Drawing for the job (mm, zero at the part's lowest x, y, z). Round coordinates to 2 decimals unless told otherwise and drop trailing zeros. Write each loop counter-clockwise with the first axis right and the second up, starting at its lowest first coordinate (ties: lowest second). Pieces come first, ordered by that corner, then holes. Notation, with made-up numbers: (13.5, 2) - (66.5, 2) arc R30 ccw to (66.5, 27) - close; hole circle Ø8 at (44, 63). An arc over 180 degrees is marked (long way). One line per question, with ' | ' between items.
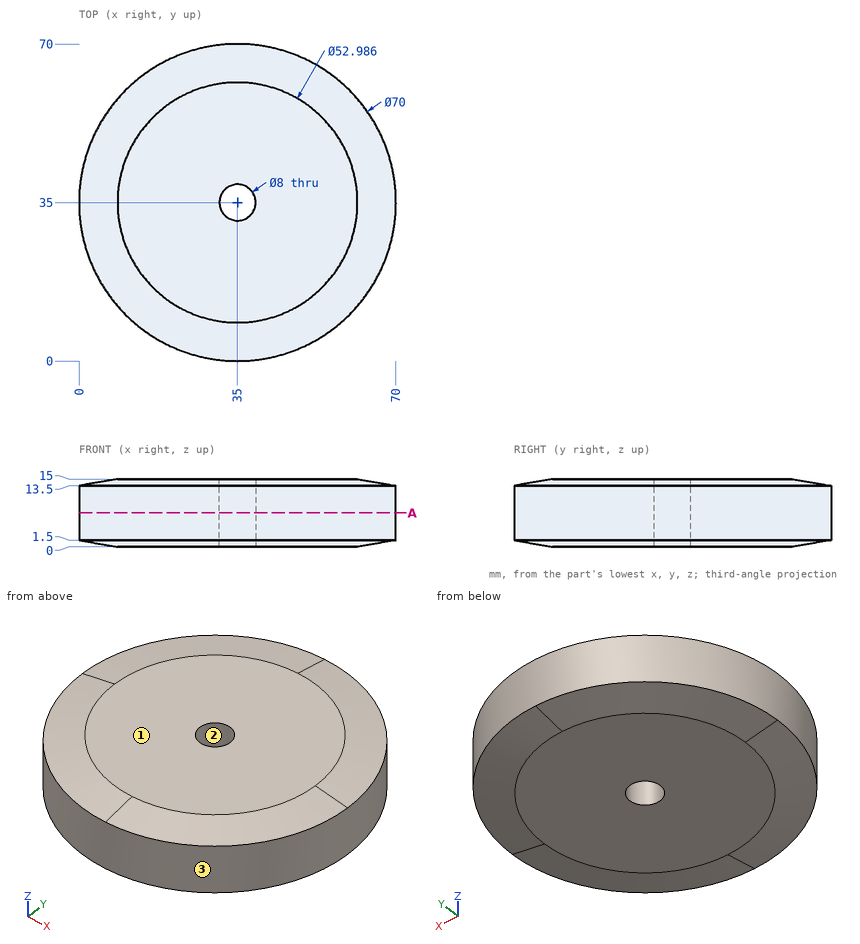
Q1. Drop flat-ended pins along their axis: pin 1 (13 mm diameter, centred on x = 35, y = 35, fed in from -Z); pin 2 (8 mm diameter, centred on x = 43, z = 2, fed in from +Y); pin 3 (2 mm diameter, centred on y = 23, z = 5, fed in from +X); pin 4 (6 mm diameter, centred on x = 47, z = 3, fed in from +Y). Give the stop position or say it passes through.
Found:
pin 1: z = 0 | pin 2: y = 69.77 | pin 3: x = 68.23 | pin 4: y = 68.82
Q2. Saw through at A-A, the plane z = 7.5. List the corners of the cut face in (x, y), then the cut area to 3 significant figures.
Found:
outline: circle Ø70 at (35, 35); hole circle Ø8 at (35, 35) | area: 3,800 mm^2
Q3. Pull direction X, two halves, no side cores. Call the marked faces 1, 2 and 3: +X half, -X half, draft (parallel to the pull), parting line (faces both ways), or undercut.
Found:
face 1: draft | face 2: undercut | face 3: parting line
Q4. Drill centre lines: L1, parallel to X at y = 38.5, z = 4.75 (1 decimal); L2, parallel to Y at x = 32.5, z = 4. Where is each one in solid material? Low to high. Write a range as from..to.
Found:
L1: 0.2..33.1, 36.9..69.8 | L2: 0.09..31.88, 38.12..69.91
